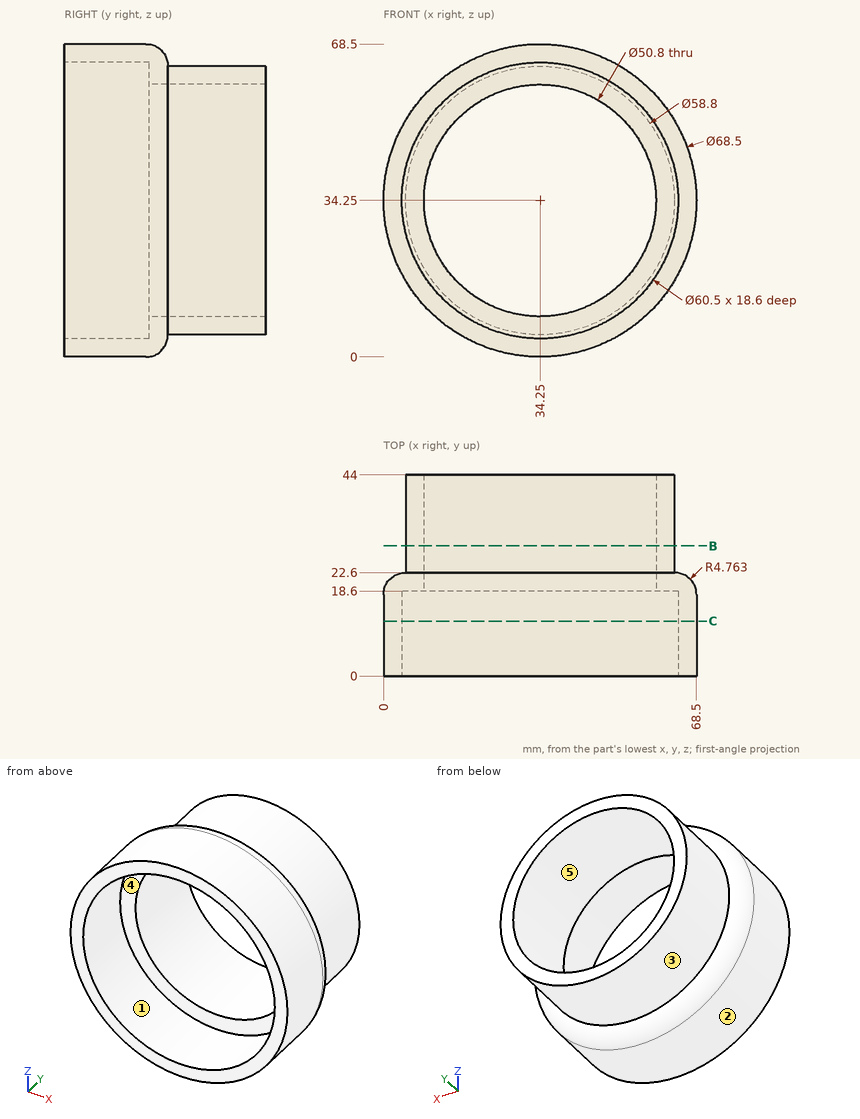
Geometry check sheet. Reference: drawing and pictorial views, mm from the part's lowest x, y, z. A direction names the side the tool comes from. Coordinates: 2 decimals unless noted, no trailing zeros. Write each loop counter-clockwise with the first axis right and the second up, starting at its lowest first coordinate (ties: lowest second). Pieces come first, ordered by that corner, then holes. Notation, with made-up numbers: (85, 3) -> (96, 3) arc R28 ccw to (96, 30) -> close; hole circle Ø9 at (55, 71). An arc over 180 degrees is marked (long way). Use a Markdown table: item, result.
1. Scan lines: line 1 along X through (y, z) = (38, 34); line 2 along Z through (x, y) = (34.25, 12.5). Record each from-to range of solid material in increasing order.
Reported:
| item | result |
|---|---|
| line 1 | x = 4.85 to 8.85, 59.65 to 63.65 |
| line 2 | z = 0 to 4, 64.5 to 68.5 |
2. Sectioned sample at B-B (y = 28.5). Enter the section's corners in (x, z).
Reported:
| item | result |
|---|---|
| outline | circle Ø58.8 at (34.25, 34.25); hole circle Ø50.8 at (34.25, 34.25) |
3. Release check for a two-part mould opening along X. For the marked faces 1 and 2 record: pulls with the +X half, pulls with the -X half, needs draft (parallel to the pull), parting line crosses it, or undercut.
Reported:
| item | result |
|---|---|
| face 1 | undercut |
| face 2 | parting line crosses it |
4. Tool access check on the marked faces 3, 4 and 5. Record the directions out of +Z, -Z, +X, -X, +Y, -Y that give a thin tool (end or side, any length) a straight path to the whole face; none if there is none.
Reported:
| item | result |
|---|---|
| face 3 | +Y |
| face 4 | -Y |
| face 5 | +Y, -Y |
5. Sectioned sample at C-C (y = 12). Enter the section's corners in (x, z).
Reported:
| item | result |
|---|---|
| outline | circle Ø68.5 at (34.25, 34.25); hole circle Ø60.5 at (34.25, 34.25) |
6. Go/stop test with flat-tipped pins: pin 1 Ø12 at (y, z) = (4.5, 61) entering from -X; pin 2 Ø12 at (y, z) = (30, 11) entering from -X; pin 3 Ø8 at (x, y) = (12, 21.5) entering from -Z; pin 4 Ø6 at (x, z) = (21.5, 17) entering from -Y. Record where each tip stops, or that it passes through.
Reported:
| item | result |
|---|---|
| pin 1 | stops at x = 7 |
| pin 2 | stops at x = 10.44 |
| pin 3 | stops at z = 5.97 |
| pin 4 | passes through |
